The listing builds one solid part. Answer for the finished solid, in the listing's coordinates (mm). A direction names the side the tool comes from. Give positions to 0.01 mm unless a question says otherwise; leave off trailing zeros. Write each loop counter-clockwise with the first axis right and the second up, starting at its lowest first coordinate (ties: lowest second). Pieces come first, ordered by that corner, then holes. Notation, with made-up numbers: (17, 60.5) - (21, 60.5) arc R17 cw to (21, 93.5) - close; hole circle Ø5 at (63, 1.25). An arc over 180 degrees is marked (long way). Answer in a Markdown table with one row per item. Add a question column.
from build123d import *

# Parameters (mm, degrees)
F1_DEPTH = 38.1
F2_DEPTH = 38.1
F0_R     = 14.2875
F3_DEPTH = 9.525


with BuildPart() as f1:
    # F0 (on Right) → F1 (new body, symmetric)
    with BuildSketch(Plane.YZ):
        Polygon((0, -254), (0, 0), (-31.75, 0), (-31.75, -31.75), (-31.75, -131.87347), (-31.75, -239.814619), (-31.75, -254), align=None)
    extrude(amount=F1_DEPTH, both=True)

    # F0 (on Right) → F2 (join, symmetric)
    with BuildSketch(Plane.YZ):
        Polygon((-31.75, -31.75), (-31.75, 0), (-190.5, 0), (-190.5, -31.75), (-177.438415, -31.75), (-101.857208, -31.75), align=None)
    extrude(amount=F2_DEPTH, both=True)

    # F0 (on Right) → F3 (join, symmetric)
    with BuildSketch(Plane.YZ):
        Polygon((-31.75, -239.814619), (-31.75, -131.87347), (-101.857208, -31.75), (-177.438415, -31.75), align=None)
        with Locations((-64.529893, -139.029505)):
            Circle(F0_R, mode=Mode.SUBTRACT)
        with Locations((-115.520839, -66.206888)):
            Circle(F0_R, mode=Mode.SUBTRACT)
    extrude(amount=F3_DEPTH, both=True)


solid = f1.part
1. Section B-B (y = -44) is taken. Give the vertices of the cut face in (x, z) (3 decimals), and give its area (3 significant figures).
2. Section C-C (x = -1.5) is taken. State how many separate pieces and enclosed holes the cut face has, and give its area (3 significant figures).
3. A tool of negligible diameter and unlimited length cuts with its end or side. For faces 1 (the face through (1, -94, 0)), 2 (the face through (0.133, -66.313, -82.513)), 3 (the face through (1, -95, -31.75)), 4 (the face through (-9.525, -89, -112)), 5 (the face through (9.525, -89, -112)), from which of +Z, -Z, +X, -X, +Y, -Y can it reach the whole face along a straight path? Write none if from no direction.
4. Section D-D (z = -59.5) is taken. Give the vertices of the cut face in (x, y) (3 decimals).
5. Straight lines are drawn through the part: L1, parallel to Z at x = -25, y = -173; L2, parallel to X at y = -82, z = -83 (3 decimals). For each, find the intervals that lie inside material, in ascending order. Write a range as [from, to].
6. Given pin 1 Ø3 at (y, z) = (-49, -181.5) entering from +X (3 decimals); pin 2 Ø12 at (x, y) = (5.5, -47.5) entering from -Z; pin 3 Ø8 at (y, z) = (-107, -81) entering from -X (3 decimals), each flat-ended and moving along its own axis, determine where each tip first touches the part or whether it passes through.
Geometry check:
| question | item | result |
|---|---|---|
| 1 | outline | (-38.1, -31.75) - (38.1, -31.75) - (38.1, 0) - (-38.1, 0) - close; (-9.525, -222.32) - (9.525, -222.32) - (9.525, -114.379) - (-9.525, -114.379) - close |
| 1 | area | 4,480 mm² |
| 2 | separate pieces | 1 |
| 2 | enclosed holes | 3 |
| 2 | area | 23,500 mm² |
| 3 | face 1 | +Z, +X, -X, +Y, -Y |
| 3 | face 2 | +X, -X |
| 3 | face 3 | none |
| 3 | face 4 | -Z, -X, -Y |
| 3 | face 5 | -Z, +X, -Y |
| 4 | outline | (-38.1, -31.75) - (38.1, -31.75) - (38.1, 0) - (-38.1, 0) - close; (-9.525, -158.008) - (9.525, -158.008) - (9.525, -128.136) - (-9.525, -128.136) - close; (-9.525, -102.905) - (9.525, -102.905) - (9.525, -82.426) - (-9.525, -82.426) - close |
| 5 | L1 | [-31.75, 0] |
| 5 | L2 | [-9.525, 9.525] |
| 6 | pin 1 | x = 9.525 |
| 6 | pin 2 | z = -225.89 |
| 6 | pin 3 | x = -9.525 |
